Design review of the part built by this model. Coordinates are the model's own, in mm. Face numbers are marked on the shaded views. A direction names the side the tool comes from. Coordinates: 2 decimals unless noted, no trailing zeros. Write each loop counter-clockwise with the first axis right and the second up, starting at its lowest first coordinate (ties: lowest second). Pieces come first, ordered by that corner, then holes.
Q1. For the marked faces 4, 5 and 6, list the 3-axis set-ups (+Z, -Z, +X, -X, +Y, -Y) from which the entire face can be reached by the end or side of a thin tool; tool diameter is ignored.
Q2. For pin 1 Ø10 at (x, y) = (61, -39) entering from +Z; pin 2 Ø17 at (y, z) = (-50.5, 167) entering from -X; pin 3 Ø1 at (y, z) = (-46.5, 170) entering from +X, all flat-tipped, find the tip position at first contact; note any pin that passes through.
Q3. Take a section at B-B, the plane y = -37. Write out the cut boundary in (x, z).
Q4. Take a section at D-D, the plane x = 182. Write out the cut boundary in (y, z), plus the area to 3 significant figures.
Q5. Take a section at C-C, the plane y = -60. Write out the cut boundary in (x, z), plus the area to 3 significant figures.
Q6. For L1, parallel to Y at x = 86, z = 239.5; L2, parallel to Z at x = 157.5, y = -61; L3, parallel to Z at x = 124.5, y = -17.5, list the stretches that pass through material, from the lowest coordinate up.
Q7. The part is to be moulded in two halves that separate along X. For the marked faces 1, 2 and 3, say which applies: released by +X, released by -X, zero draft, split by the parting line, or undercut.
Q8. Take a section at A-A, the plane x = 109.5. Write out the cut boundary in (y, z), plus the area to 3 significant figures.
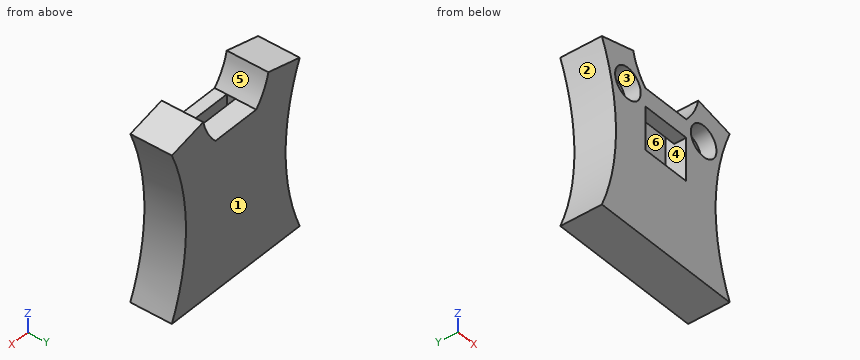
from build123d import *

# Parameters (mm, degrees)
F1_DEPTH = 67
F2_W     = 40
F2_H     = 69.649726
F3_DEPTH = 28
F2_R     = 25
F4_DEPTH = 25
F5_W     = 80
F5_H     = 14
F6_DEPTH = 100


with BuildPart() as f1:
    # F0 (on Front) → F1 (new body)
    with BuildSketch(Plane.XZ):
        with BuildLine():
            ThreePointArc((0, 270), (27.477124, 135), (0, 0))
            Line((0, 0), (125, 0))
            Line((125, 0), (125, 240))
            Line((125, 240), (85, 240))
            ThreePointArc((85, 240), (70.310796, 261.057784), (61.28452, 285.093784))
            Line((61.28452, 285.093784), (0, 270))
        make_face()
        with BuildLine():
            Line((125, 240), (125, 0))
            Line((125, 0), (250, 0))
            ThreePointArc((250, 0), (222.522876, 135), (250, 270))
            Line((250, 270), (188.71548, 285.093784))
            ThreePointArc((188.71548, 285.093784), (179.689204, 261.057784), (165, 240))
            Line((165, 240), (125, 240))
        make_face()
    extrude(amount=F1_DEPTH)

    # F2 (on face) → F3 (cut)
    with BuildSketch(Plane.XZ.offset(67)):
        with Locations((105, 175.762683)):
            Rectangle(F2_W, F2_H)
        with Locations((145, 175.762683)):
            Rectangle(F2_W, F2_H)
    extrude(amount=-F3_DEPTH, mode=Mode.SUBTRACT)

    # F2 (on face) → F4 (cut)
    with BuildSketch(Plane.XZ.offset(67)):
        with Locations((105, 175.762683)):
            Rectangle(F2_W, F2_H)
        with Locations((145, 175.762683)):
            Rectangle(F2_W, F2_H)
        with Locations((50.898362, 226.223186)):
            Circle(F2_R)
        with Locations((199.101638, 226.223186)):
            Circle(F2_R)
    extrude(amount=-F4_DEPTH, mode=Mode.SUBTRACT)

    # F5 (on face) → F6 (cut)
    with BuildSketch(Plane.XY.offset(240)):
        with Locations((125, -40.5)):
            Rectangle(F5_W, F5_H)
    extrude(amount=-F6_DEPTH, mode=Mode.SUBTRACT)


solid = f1.part
Responses:
1. face 4: none
1. face 5: +Z, +Y, -Y
1. face 6: +Z
2. pin 1: stops at z = 285.09
2. pin 2: stops at x = 25.09
2. pin 3: stops at x = 224.35
3. outline: (0, 0) - (250, 0) arc R345.38 cw to (250, 270) - (188.72, 285.09) arc R103.03 cw to (165, 240) - (165, 140) - (85, 140) - (85, 240) arc R103.03 cw to (61.28, 285.09) - (0, 270) arc R345.38 cw to start
4. outline: (-67, 0) - (0, 0) - (0, 265.74) - (-67, 265.74) - (-67, 244.46) - (-42, 244.46) - (-42, 207.99) - (-67, 207.99) - close
4. area: 16,900 mm2
5. outline: (0, 0) - (250, 0) arc R345.38 cw to (250, 270) - (188.72, 285.09) arc R103.03 cw to (165, 240) - (85, 240) arc R103.03 cw to (61.28, 285.09) - (0, 270) arc R345.38 cw to start; hole circle Ø50 at (50.9, 226.22); hole (85, 140.94) - (165, 140.94) - (165, 210.59) - (85, 210.59) - close; hole circle Ø50 at (199.1, 226.22)
5. area: 46,000 mm2
6. L1: y = -67 to -47.5, -33.5 to 0
6. L2: z = 0 to 140.94, 210.59 to 240
6. L3: z = 0 to 240
7. face 1: zero draft
7. face 2: released by -X
7. face 3: undercut
8. outline: (-67, 0) - (0, 0) - (0, 240) - (-33.5, 240) - (-33.5, 140) - (-47.5, 140) - (-47.5, 140.94) - (-67, 140.94) - close; (-67, 210.59) - (-47.5, 210.59) - (-47.5, 240) - (-67, 240) - close
8. area: 13,300 mm2
